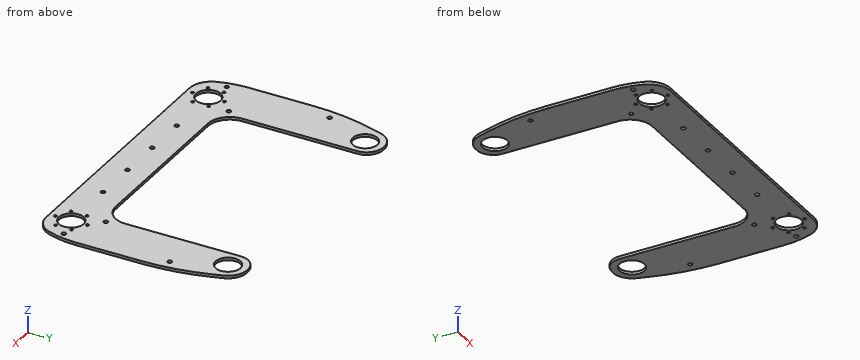
from build123d import *

# Parameters (mm, degrees)
SKETCH1_R           = 14.2875
SKETCH1_R_2         = 1.6002
SKETCH1_R_3         = 2.4892
BOSS_EXTRUDE3_DEPTH = 3.175
SKETCH2_W           = 355.6
SKETCH2_H           = 19.05
CUT_EXTRUDE1_DEPTH  = 290.621961572
FILLET1_R           = 19.05
CUT_EXTRUDE2_DEPTH  = 290.621961572
FILLET2_R           = 254
FILLET3_R           = 254
CUT_EXTRUDE3_DEPTH  = 290.621961572
FILLET4_R           = 25.4


with BuildPart() as part:
    # Sketch1 → Boss-Extrude3 (new body)
    with BuildSketch(Plane.XY):
        with BuildLine():
            Line((120.65, -152.4), (120.65, -6.35))
            Line((120.65, -6.35), (120.65, 6.35))
            ThreePointArc((120.65, 6.35), (124.369743879, 15.330256121), (133.35, 19.05))
            Line((133.35, 19.05), (165.1, 19.05))
            ThreePointArc((165.1, 19.05), (174.080256121, 15.330256121), (177.8, 6.35))
            Line((177.8, 6.35), (177.8, -6.35))
            Line((177.8, -6.35), (177.8, -222.25))
            ThreePointArc((177.8, -222.25), (175.940128061, -226.740128061), (171.45, -228.6))
            Line((171.45, -228.6), (12.7, -228.6))
            Line((12.7, -228.6), (-12.7, -228.6))
            Line((-12.7, -228.6), (-171.45, -228.6))
            ThreePointArc((-171.45, -228.6), (-175.940128061, -226.740128061), (-177.8, -222.25))
            Line((-177.8, -222.25), (-177.8, -6.35))
            Line((-177.8, -6.35), (-177.8, 6.35))
            ThreePointArc((-177.8, 6.35), (-174.080256121, 15.330256121), (-165.1, 19.05))
            Line((-165.1, 19.05), (-133.35, 19.05))
            ThreePointArc((-133.35, 19.05), (-124.369743879, 15.330256121), (-120.65, 6.35))
            Line((-120.65, 6.35), (-120.65, -6.35))
            Line((-120.65, -6.35), (-120.65, -152.4))
            ThreePointArc((-120.65, -152.4), (-113.210512242, -170.360512242), (-95.25, -177.8))
            Line((-95.25, -177.8), (-12.7, -177.8))
            Line((-12.7, -177.8), (12.7, -177.8))
            Line((12.7, -177.8), (95.25, -177.8))
            ThreePointArc((95.25, -177.8), (113.210512242, -170.360512242), (120.65, -152.4))
        make_face()
        with Locations((141.605, -22.02688)):
            Circle(SKETCH1_R, mode=Mode.SUBTRACT)
        with Locations(Location((-141.605, -22.02688, 0), (0, 0, 180))):
            Circle(SKETCH1_R, mode=Mode.SUBTRACT)
        with Locations((-141.605, -203.2)):
            Circle(SKETCH1_R, mode=Mode.SUBTRACT)
        with Locations((-141.605, -184.724802)):
            Circle(SKETCH1_R_2, mode=Mode.SUBTRACT)
        with Locations((-125.604004596, -193.962981004)):
            Circle(SKETCH1_R_2, mode=Mode.SUBTRACT)
        with Locations((-125.604004596, -212.439339011)):
            Circle(SKETCH1_R_2, mode=Mode.SUBTRACT)
        with Locations((-141.605, -221.677518015)):
            Circle(SKETCH1_R_2, mode=Mode.SUBTRACT)
        with Locations((-157.605995404, -212.439339011)):
            Circle(SKETCH1_R_2, mode=Mode.SUBTRACT)
        with Locations((-157.605995404, -193.962981004)):
            Circle(SKETCH1_R_2, mode=Mode.SUBTRACT)
        with Locations(Location((157.605995404, -212.439339011, 0), (0, 0, 180))):
            Circle(SKETCH1_R_2, mode=Mode.SUBTRACT)
        with Locations(Location((157.605995404, -193.962981004, 0), (0, 0, 180))):
            Circle(SKETCH1_R_2, mode=Mode.SUBTRACT)
        with Locations(Location((141.605, -184.724802, 0), (0, 0, 180))):
            Circle(SKETCH1_R_2, mode=Mode.SUBTRACT)
        with Locations(Location((125.604004596, -193.962981004, 0), (0, 0, 180))):
            Circle(SKETCH1_R_2, mode=Mode.SUBTRACT)
        with Locations(Location((125.604004596, -212.439339011, 0), (0, 0, 180))):
            Circle(SKETCH1_R_2, mode=Mode.SUBTRACT)
        with Locations(Location((141.605, -221.677518015, 0), (0, 0, 180))):
            Circle(SKETCH1_R_2, mode=Mode.SUBTRACT)
        with Locations(Location((141.605, -203.2, 0), (0, 0, 180))):
            Circle(SKETCH1_R, mode=Mode.SUBTRACT)
        with Locations((-76.2, -203.2)):
            Circle(SKETCH1_R_3, mode=Mode.SUBTRACT)
        with Locations(Location((76.2, -203.2, 0), (0, 0, 180))):
            Circle(SKETCH1_R_3, mode=Mode.SUBTRACT)
        with Locations((-25.4, -203.2)):
            Circle(SKETCH1_R_3, mode=Mode.SUBTRACT)
        with Locations((-127, -171.45)):
            Circle(SKETCH1_R_3, mode=Mode.SUBTRACT)
        with Locations((-149.225, 6.35)):
            Circle(SKETCH1_R_3, mode=Mode.SUBTRACT)
        with Locations(Location((127, -171.45, 0), (0, 0, 180))):
            Circle(SKETCH1_R_3, mode=Mode.SUBTRACT)
        with Locations(Location((149.225, 6.35, 0), (0, 0, 180))):
            Circle(SKETCH1_R_3, mode=Mode.SUBTRACT)
        with Locations((-168.275, -196.85)):
            Circle(SKETCH1_R_3, mode=Mode.SUBTRACT)
        with Locations(Location((168.275, -196.85, 0), (0, 0, 180))):
            Circle(SKETCH1_R_3, mode=Mode.SUBTRACT)
        with Locations((-165.1, -76.2)):
            Circle(SKETCH1_R_3, mode=Mode.SUBTRACT)
        with Locations(Location((165.1, -76.2, 0), (0, 0, 180))):
            Circle(SKETCH1_R_3, mode=Mode.SUBTRACT)
        with Locations(Location((25.4, -203.2, 0), (0, 0, 180))):
            Circle(SKETCH1_R_3, mode=Mode.SUBTRACT)
    extrude(amount=BOSS_EXTRUDE3_DEPTH)

    # Sketch2 → Cut-Extrude1 (cut, through all)
    with BuildSketch(Plane.XY.offset(3.175)):
        with Locations((0, 9.525)):
            Rectangle(SKETCH2_W, SKETCH2_H)
    extrude(amount=-CUT_EXTRUDE1_DEPTH, mode=Mode.SUBTRACT)

    # Fillet1
    fillet1_edges = [part.edges().sort_by_distance(p)[0] for p in [
        (-177.8, 0, 1.5875),
        (120.65, 0, 1.5875),
        (177.8, 0, 1.5875),
        (-120.65, 0, 1.5875),
    ]]
    fillet(fillet1_edges, radius=FILLET1_R)

    # Sketch3 → Cut-Extrude2 (cut, through all)
    with BuildSketch(Plane.XY.offset(3.175)):
        with BuildLine():
            Line((-177.8, 0), (-177.8, -63.5))
            Line((-177.8, -63.5), (-162.698792053, -15.403859213))
            ThreePointArc((-162.698792053, -15.403859213), (-155.445369527, -4.785747819), (-143.51, 0))
            Line((-143.51, 0), (-177.8, 0))
        make_face()
    cut_extrude2 = extrude(amount=-CUT_EXTRUDE2_DEPTH, mode=Mode.SUBTRACT)

    # Mirror1: Cut-Extrude2 across plane
    add(cut_extrude2.mirror(Plane(origin=(0, 0, 0), x_dir=(0, 0, 1), z_dir=(1, 0, 0))), mode=Mode.SUBTRACT)

    # Fillet2
    fillet2_edges = [part.edges().sort_by_distance(p)[0] for p in [
        (-177.8, -63.5, 1.5875),
    ]]
    fillet(fillet2_edges, radius=FILLET2_R)

    # Fillet3
    fillet3_edges = [part.edges().sort_by_distance(p)[0] for p in [
        (177.8, -63.5, 1.5875),
    ]]
    fillet(fillet3_edges, radius=FILLET3_R)

    # Sketch4 → Cut-Extrude3 (cut, through all)
    with BuildSketch(Plane.XY.offset(3.175)):
        with BuildLine():
            ThreePointArc((-164.188181024, -228.6), (-174.338063951, -204.096014982), (-177.8, -177.8))
            Line((-177.8, -177.8), (-177.8, -222.25))
            ThreePointArc((-177.8, -222.25), (-175.940128061, -226.740128061), (-171.45, -228.6))
            Line((-171.45, -228.6), (-164.188181024, -228.6))
        make_face()
        with BuildLine():
            ThreePointArc((177.8, -177.8), (174.338063951, -204.096014982), (164.188181024, -228.6))
            Line((164.188181024, -228.6), (171.45, -228.6))
            ThreePointArc((171.45, -228.6), (175.940128061, -226.740128061), (177.8, -222.25))
            Line((177.8, -222.25), (177.8, -177.8))
        make_face()
    extrude(amount=-CUT_EXTRUDE3_DEPTH, mode=Mode.SUBTRACT)

    # Fillet4
    fillet4_edges = [part.edges().sort_by_distance(p)[0] for p in [
        (-164.188181024, -228.6, 1.5875),
        (164.188181024, -228.6, 1.5875),
    ]]
    fillet(fillet4_edges, radius=FILLET4_R)


solid = part.part
Design review of the part built by this model. Coordinates are the model's own, in mm. Coordinates: 2 decimals unless noted, no trailing zeros. Loops run counter-clockwise (first coordinate to the right, second up) from the corner with the lowest first, then second, coordinate; pieces in that order, holes last. Notation, with made-up numbers: (31.25, 53) -> (37.25, 53) arc R15 cw to (37.25, 60) -> close; hole circle Ø7 at (63, 58). An arc over 180 degrees is marked (long way). Use a Markdown table: item, result. Add a question column.
Item 1: Clearance check with a flat-ended pin moving along its axis: P1, Ø3, axis at x = 157.61, y = -212.44, coming from the -Z side. State where the tip first meets the part, or that it passes through.
Item 2: We need section A-A, the plane y = -137. Write out the cut boundary in (x, z) (3 decimals).
Item 3: We need section C-C, the plane x = 88.5. Write out the cut boundary in (y, z) (3 decimals), and give its area (3 significant figures).
Item 4: We need section B-B, the plane x = 135.5. Write out the cut boundary in (y, z) (1 decimal), and give its area (3 significant figures).
Item 5: We need section D-D, the plane z = 0.95. Count the separate pieces of the cut face and the enclosed holes in it, and give its area (3 significant figures).
Item 6: Wall thickness on L1, parallel to X at y = -35, z = 3; L2, parallel to X at y = -138, z = 2.4; L3, parallel to X at y = -207, z = 1.25: over which ranges is each line inside the solid? List them lowest first. Write a range as from..to.
Numbers:
| question | item | result |
|---|---|---|
| 1 | P1 | passes through |
| 2 | outline | (-177.8, 0) -> (-120.65, 0) -> (-120.65, 3.175) -> (-177.8, 3.175) -> close; (120.65, 0) -> (177.8, 0) -> (177.8, 3.175) -> (120.65, 3.175) -> close |
| 3 | outline | (-228.6, 0) -> (-177.8, 0) -> (-177.8, 3.175) -> (-228.6, 3.175) -> close |
| 3 | area | 161 mm^2 |
| 4 | outline | (-228.6, 0) -> (-216.1, 0) -> (-216.1, 3.2) -> (-228.6, 3.2) -> close; (-190.3, 0) -> (-34.9, 0) -> (-34.9, 3.2) -> (-190.3, 3.2) -> close; (-9.1, 0) -> (-0.5, 0) -> (-0.5, 3.2) -> (-9.1, 3.2) -> close |
| 4 | area | 560 mm^2 |
| 5 | separate pieces | 1 |
| 5 | enclosed holes | 26 |
| 5 | area | 33,600 mm^2 |
| 6 | L1 | x = -168.68..-147.59, -135.62..-120.65, 120.65..135.62, 147.59..168.68 |
| 6 | L2 | x = -177.8..-120.65, 120.65..177.8 |
| 6 | L3 | x = -173.51..-155.38, -127.83..127.83, 155.38..173.51 |
